Geometry: final body of the model. Coordinates: model frame, mm. A direction names the side the tool comes from. Give positions to 0.01 mm unless a question says otherwise; leave off trailing zeros. Write each loop counter-clockwise with the first axis right and the second up, starting at its lowest first coordinate (ties: lowest second). Pieces come first, ordered by that corner, then holes. Notation, with made-up numbers: M 48,10.25 L 59,10.25 A11 cw 59,31.25 Z; hole C -22.5,26 d11. An arc over 180 degrees is marked long. Use a Markdown table: item, result. Add a question column.
1) Section A-A on y = 8. Return the cut outline in (x, z).
2) Pin query (flat end, axial travel): pin 1 (2 mm diameter, centred on x = -11, z = 0, fed in from +Y); pin 2 (1.5 mm diameter, centred on x = 11, z = 0, fed in from -Y). Return the tip coordinate at first contact, or that it passes through.
3) Section C-C on x = -3.75. Return the cut outline in (y, z).
4) Section D-D on z = -2.35. State how many separate pieces and enclosed holes the cut face has, then the cut area to 3 significant figures.
5) Line query: line 1 (Y direction, x = 11.5, z = 1.7); line 2 (Y direction, x = 4.5, z = -2.5); line 3 (X direction, y = -17, z = -0.05). Output: solid intervals per line, ascending.
6) Draft query along X for faces 4 (the cylindrical face through (-11.13, -5.71, 0.04)), 5 (the cylindrical face through (13.699, -18.665, 0.042)), 6 (the cylindrical face through (-13.715, 18.649, -0.042)), 7 (the flat face through (0, 18.95, 0)). Return one class per face: +X half, -X half, draft (parallel to the pull), parting line (faces both ways), or undercut.
7) Set-up query: faces 1 (the cylindrical face through (-12.24, 15.75, -0.16)), 2 (the cylindrical face through (-7.4, 15.38, 0.04)), 3 (the flat face through (14, 0, 0)). Return all of +Z, -Z, +X, -X, +Y, -Y with unobstructed straight access to the full face (end or side cutting, diameter ignored); none if empty.
8) Section B-B on y = -5. Return the cut outline in (x, z).
```python
from build123d import *
from OCP.BRepFilletAPI import BRepFilletAPI_MakeFillet

# Parameters (mm, degrees)
SKETCH_1_W                  = 28
SKETCH_1_H                  = 37.9
EXTRUDE_1_DEPTH             = 3
HOLE_WIZARD_M3_1_AT_2_COUNT = 2
HOLE_WIZARD_M3_1_AT_2_PITCH = 22
HOLE_WIZARD_M2_1_D          = 1.6
SKETCH_8_W                  = 16
SKETCH_8_H                  = 31.9
CUT_EXTRUDE_1_DEPTH         = 18
SKETCH_9_W                  = 19
SKETCH_9_H                  = 23.9
CUT_EXTRUDE_2_DEPTH         = 18
FILLET_1_R                  = 2
FILLET_2_R1                 = 2
FILLET_2_R2                 = 1


with BuildPart() as part:
    # 草图1 → 凸台-拉伸1 (new, symmetric)
    with BuildSketch(Plane.XY):
        Rectangle(SKETCH_1_W, SKETCH_1_H)
    extrude(amount=EXTRUDE_1_DEPTH, both=True)

    # 草图4 → M3 螺纹孔1 (revolve, cut)
    with BuildSketch(Plane(origin=(-11, 18.95, 0), x_dir=(0, 0, 1), z_dir=(1, 0, 0))):
        Polygon((0, 0), (0, 7.251075774), (1.25, 6.5), (1.25, 0), align=None)
    hole_wizard_m3_1 = revolve(axis=Axis((-11, 25.3, 0), (0, -1, 0)), mode=Mode.SUBTRACT)

    # M3 螺纹孔1 at 2: M3 螺纹孔1 ×2
    with Locations(*[(i * HOLE_WIZARD_M3_1_AT_2_PITCH, 0, 0) for i in range(1, HOLE_WIZARD_M3_1_AT_2_COUNT)]):
        add(hole_wizard_m3_1, mode=Mode.SUBTRACT)

    # 镜向1: M3 螺纹孔1 across plane
    add(hole_wizard_m3_1.mirror(Plane.ZX), mode=Mode.SUBTRACT)

    # 镜向1 copy 1 sketch → 镜向1 copy 1 (revolve, cut)
    with BuildSketch(Plane(origin=(11, -18.95, 0), x_dir=(0, 0, 1), z_dir=(1, 0, 0))):
        Polygon((0, 0), (0, -7.251075774), (1.25, -6.5), (1.25, 0), align=None)
    revolve(axis=Axis((11, -25.3, 0), (0, -1, 0)), mode=Mode.SUBTRACT)

    # M2 螺纹孔1 (through all)
    with Locations(Plane(origin=(0, 0, -3), x_dir=(-1, 0, 0), z_dir=(0, 0, -1))):
        with Locations((-11.5, 10), (11.5, 10), (11.5, -5), (-11.5, -5)):
            Hole(HOLE_WIZARD_M2_1_D / 2)

    # 草图8 → 切除-拉伸1 (cut, symmetric)
    with BuildSketch(Plane(origin=(0, 0, -3), x_dir=(-1, 0, 0), z_dir=(0, 0, -1))):
        Rectangle(SKETCH_8_W, SKETCH_8_H)
    extrude(amount=CUT_EXTRUDE_1_DEPTH, both=True, mode=Mode.SUBTRACT)

    # 草图9 → 切除-拉伸2 (cut, symmetric)
    with BuildSketch(Plane(origin=(0, 0, -3), x_dir=(-1, 0, 0), z_dir=(0, 0, -1))):
        Rectangle(SKETCH_9_W, SKETCH_9_H)
    extrude(amount=CUT_EXTRUDE_2_DEPTH, both=True, mode=Mode.SUBTRACT)

    # 圆角1
    # the kernel refuses this fillet: 2 mm, written as the material it adds along each edge
    with BuildSketch(Plane(origin=(-9.5, 11.95, 3), x_dir=(1, 0, 0), z_dir=(0, 0, -1))) as fillet_1_piece_1:
        with BuildLine():
            CenterArc((2, 1.936491673), FILLET_1_R, 180, 75.522487814)
            Line((0, 1.936491673), (-0.04, 1.936491673))
            Line((-0.04, 1.936491673), (-0.04, 0))
            Line((-0.04, 0), (0, -0.04))
            ThreePointArc((0, -0.04), (0.75, -0.04), (1.49, -0.038729833))
            Line((1.49, -0.038729833), (1.5, 0))
        make_face()
    extrude(amount=6)
    with BuildSketch(Plane(origin=(-9.5, -11.95, 3), x_dir=(0, 1, 0), z_dir=(0, 0, -1))) as fillet_1_piece_2:
        with BuildLine():
            CenterArc((1.936491673, 2), FILLET_1_R, 194.477512186, 75.522487814)
            Line((0, 1.5), (-0.038729833, 1.49))
            ThreePointArc((-0.038729833, 1.49), (-0.04, 0.75), (-0.04, 0))
            Line((-0.04, 0), (0, -0.04))
            Line((0, -0.04), (1.936491673, -0.04))
            Line((1.936491673, -0.04), (1.936491673, 0))
        make_face()
    extrude(amount=6)
    with BuildSketch(Plane(origin=(9.5, -11.95, -3), x_dir=(-1, 0, 0), z_dir=(0, 0, 1))) as fillet_1_piece_3:
        with BuildLine():
            CenterArc((2, -1.936491673), FILLET_1_R, 104.477512186, 75.522487814)
            Line((0, -1.936491673), (-0.04, -1.936491673))
            Line((-0.04, -1.936491673), (-0.04, 0))
            Line((-0.04, 0), (0, 0.04))
            ThreePointArc((0, 0.04), (0.75, 0.04), (1.49, 0.038729833))
            Line((1.49, 0.038729833), (1.5, 0))
        make_face()
    extrude(amount=6)
    with BuildSketch(Plane(origin=(9.5, 11.95, -3), x_dir=(0, -1, 0), z_dir=(0, 0, 1))) as fillet_1_piece_4:
        with BuildLine():
            CenterArc((1.936491673, -2), FILLET_1_R, 90, 75.522487814)
            Line((0, -1.5), (-0.038729833, -1.49))
            ThreePointArc((-0.038729833, -1.49), (-0.04, -0.75), (-0.04, 0))
            Line((-0.04, 0), (0, 0.04))
            Line((0, 0.04), (1.936491673, 0.04))
            Line((1.936491673, 0.04), (1.936491673, 0))
        make_face()
    extrude(amount=6)

    # 圆角2: one fillet with a radius per group of edges: ONE call of the kernel's fillet builder (fillet() takes one radius for all edges)
    fillet_2_edges_1 = [part.edges().sort_by_distance(p)[0] for p in [
        (8, 11.95, 0),
        (8, 15.95, 0),
        (-8, -11.95, 0),
        (-8, 11.95, 0),
        (-8, 15.95, 0),
        (8, -11.95, 0),
        (8, -15.95, 0),
        (-8, -15.95, 0),
    ]]
    fillet_2_edges_2 = [part.edges().sort_by_distance(p)[0] for p in [
        (14, 18.95, 0),
        (-14, 18.95, 0),
        (-14, -18.95, 0),
        (14, -18.95, 0),
    ]]
    fillet_2 = BRepFilletAPI_MakeFillet(part.part.solid().wrapped)
    for e in fillet_2_edges_1:
        fillet_2.Add(FILLET_2_R1, e.wrapped)
    for e in fillet_2_edges_2:
        fillet_2.Add(FILLET_2_R2, e.wrapped)
    add(Compound.cast(fillet_2.Shape()), mode=Mode.REPLACE)


solid = part.part
```
Found:
| question | item | result |
|---|---|---|
| 1 | outline | M -14,-3 L -9.5,-3 L -9.5,3 L -14,3 Z; M 9.5,-3 L 14,-3 L 14,3 L 9.5,3 Z |
| 2 | pin 1 | y = 12.3 |
| 2 | pin 2 | y = -12.15 |
| 3 | outline | M -18.95,-3 L -15.95,-3 L -15.95,3 L -18.95,3 Z; M 15.95,-3 L 18.95,-3 L 18.95,3 L 15.95,3 Z |
| 4 | separate pieces | 1 |
| 4 | enclosed holes | 5 |
| 4 | area | 476 mm² |
| 5 | line 1 | -18.95 to -5.8, -4.2 to 9.2, 10.8 to 18.95 |
| 5 | line 2 | -18.95 to -15.95, 15.95 to 18.95 |
| 5 | line 3 | -14 to -12.25, -9.75 to 9.75, 12.25 to 14 |
| 6 | face 4 | undercut |
| 6 | face 5 | +X half |
| 6 | face 6 | -X half |
| 6 | face 7 | draft |
| 7 | face 1 | +Y |
| 7 | face 2 | +Z, -Z |
| 7 | face 3 | +Z, -Z, +X, +Y, -Y |
| 8 | outline | M -14,-3 L -12.3,-3 L -12.3,3 L -14,3 Z; M -10.7,-3 L -9.5,-3 L -9.5,3 L -10.7,3 Z; M 9.5,-3 L 10.7,-3 L 10.7,3 L 9.5,3 Z; M 12.3,-3 L 14,-3 L 14,3 L 12.3,3 Z |
